```python
from build123d import *

# Parameters (mm, degrees)
EXTRUDE_1_DEPTH     = 10
CUT_EXTRUDE_2_DEPTH = 1.5


with BuildPart() as part:
    # 草图1 → 旋转1 (revolve)
    with BuildSketch(Plane.XY, mode=Mode.PRIVATE) as revolve_1_sk:
        Polygon((0, 0), (0, 2.5), (0.5, 3), (3.5, 3), (3.5, 3.9), (3.6, 4), (13.5, 4), (13.5, 5.9), (13.6, 6), (15, 6), (15, 0), align=None)
    revolve(revolve_1_sk.sketch.rotate(Axis((15, 0, 0), (-1, 0, 0)), 90), axis=Axis((15, 0, 0), (-1, 0, 0)))

    # 草图2 → 凸台-拉伸1 (add)
    with BuildSketch(Plane(origin=(15, 0, 0), x_dir=(0, 0, -1), z_dir=(1, 0, 0))):
        with BuildLine():
            Line((-3.565863992, 4.065863992), (3.565863992, 4.065863992))
            ThreePointArc((3.565863992, 4.065863992), (3.919417382, 3.919417382), (4.065863992, 3.565863992))
            Line((4.065863992, 3.565863992), (4.065863992, -3.565863992))
            ThreePointArc((4.065863992, -3.565863992), (3.919417382, -3.919417382), (3.565863992, -4.065863992))
            Line((3.565863992, -4.065863992), (-3.565863992, -4.065863992))
            ThreePointArc((-3.565863992, -4.065863992), (-3.919417382, -3.919417382), (-4.065863992, -3.565863992))
            Line((-4.065863992, -3.565863992), (-4.065863992, 3.565863992))
            ThreePointArc((-4.065863992, 3.565863992), (-3.919417382, 3.919417382), (-3.565863992, 4.065863992))
        make_face()
    extrude(amount=EXTRUDE_1_DEPTH)

    # 草图3 → 切除-拉伸2 (cut)
    with BuildSketch(Plane(origin=(25, 0, 0), x_dir=(0, 0, -1), z_dir=(1, 0, 0))):
        Polygon((-4.065863992, 3.565863992), (-3.565863992, 4.065863992), (-4.065863992, 4.065863992), align=None)
        Polygon((3.565863992, 4.065863992), (4.065863992, 3.565863992), (4.065863992, 4.065863992), align=None)
        Polygon((-4.065863992, -3.565863992), (-3.565863992, -4.065863992), (-4.065863992, -4.065863992), align=None)
        Polygon((3.565863992, -4.065863992), (4.065863992, -3.565863992), (4.065863992, -4.065863992), align=None)
    extrude(amount=-CUT_EXTRUDE_2_DEPTH, mode=Mode.SUBTRACT)

    # 草图5 → 旋转2 (revolve)
    with BuildSketch(Plane.XY, mode=Mode.PRIVATE) as revolve_2_sk:
        Polygon((35, 3.9), (35, 3), (38, 3), (38.5, 2.5), (38.5, 0), (25, 0), (25, 4), (34.9, 4), align=None)
    revolve(revolve_2_sk.sketch.rotate(Axis((38.5, 0, 0), (-1, 0, 0)), 90), axis=Axis((38.5, 0, 0), (-1, 0, 0)))


solid = part.part
```
CAD build for the part. Positions are in the model's coordinates, mm. A direction names the side the tool comes from. Give positions to 0.01 mm unless a question says otherwise; leave off trailing zeros. Write each loop counter-clockwise with the first axis right and the second up, starting at its lowest first coordinate (ties: lowest second). Pieces come first, ordered by that corner, then holes. Notation, with made-up numbers: (-21, 77) -> (30, 77) arc R9 cw to (30, 87) -> close; hole circle Ø5 at (-1.5, 59). An arc over 180 degrees is marked (long way). Write each question's results on one line, items separated by ' | '.
1. Which spindle directions (+Z, -Z, +X, -X, +Y, -Y) get a long thin tool onto all of the face, cutting with end or side? Do faces 1 (the flat face through (35, 3, -1)), 2 (the flat face through (20, 4.066, 0)), 3 (the cylindrical face through (8.619, 3.905, 0.867)), 4 (the flat face through (20, 0, -4.066)). Say none if no direction does.
Geometry check:
face 1: +X | face 2: +Z, -Z, +X, +Y | face 3: -X | face 4: -Z, +X, +Y, -Y
2. Wall check: probe 1 along Z at (x, y) = (22, -1); probe 2 along Z at (x, y) = (14.5, 0.25); probe 3 along X at (y, z) = (-2, -5.5). Give the ranges that are in metal, low to high. Write a range as [from, to].
Geometry check:
probe 1: [-4.07, 4.07] | probe 2: [-5.99, 5.99] | probe 3: [13.5, 15]
3. Drop flat-ended pins along their axis: P1, Ø2, axis at x = 31.5, y = 0.5, coming from the -Z side; P2, Ø2, axis at x = 20, z = 0, coming from the +Y side; P3, Ø3.5, axis at x = 22, y = -1, coming from the +Z side. Give the stop position or say it passes through.
Geometry check:
P1: z = -4 | P2: y = 4.07 | P3: z = 4.07
4. Cut at A-A, the plane x = 17. Write the cut outline in (y, z), then the cut area to 3 significant figures.
Geometry check:
outline: (-4.07, -3.57) arc R0.5 ccw to (-3.57, -4.07) -> (3.57, -4.07) arc R0.5 ccw to (4.07, -3.57) -> (4.07, 3.57) arc R0.5 ccw to (3.57, 4.07) -> (-3.57, 4.07) arc R0.5 ccw to (-4.07, 3.57) -> close | area: 65.9 mm²
5. Cut at D-D, the plane x = 9.5. Write the cut outline in (y, z).
Geometry check:
outline: circle Ø8 at (0, 0)
